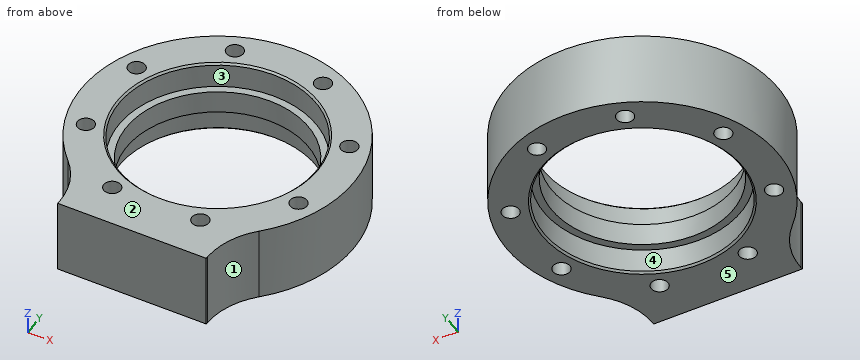
Autodesk Inventor part; units mm, degrees
ref_plane "YZ Plane" through (0, 0, 0) normal (1, 0, 0) x (0, 1, 0)
ref_plane "XZ Plane" through (0, 0, 0) normal (0, 1, 0) x (-1, 0, 0)
ref_plane "XY Plane" through (0, 0, 0) normal (0, 0, 1) x (1, 0, 0)
sketch "スケッチ1" plane through (0, 0, 0) normal (1, 0, 0) x (0, 1, 0)
  line L0 (26.1, 0) -> (36.1, 0)
  line L1 (36.1, 0) -> (36.1, 20)
  line L2 (36.1, 20) -> (26.1, 20)
  line L3 (26.1, 20) -> (26.1, 13.05)
  line L4 (26.1, 13.05) -> (24.1, 13.05)
  line L5 (0, -4) -> (0, 24)
  line L6 (24.1, 13.05) -> (24.1, 6.95)
  line L7 (24.1, 6.95) -> (26.1, 6.95)
  line L8 (26.1, 6.95) -> (26.1, 0)
  point P0 (0, 0)
  dimension "d0" = 26.1
  dimension "d2" = 6.95
  dimension "d3" = 20
  dimension "d4" = 10
  dimension "d28" = 2
  dimension "d29" = 6.95
revolve "回転1" add sketch "スケッチ1" angle 360 about axis through (0, 0, -10) along (0, 0, 1)
sketch "スケッチ2" plane through (0, 0, 0) normal (0, 0, -1) x (-1, 0, 0)
  circle A0 centre (0, 0) radius 31
  point P0 (-11.8632, 28.6403)
  point P1 (-28.6403, 11.8632)
  point P2 (-28.6403, -11.8632)
  point P3 (-11.8632, -28.6403)
  point P4 (11.8632, -28.6403)
  point P5 (28.6403, -11.8632)
  point P6 (28.6403, 11.8632)
  point P7 (11.8632, 28.6403)
  dimension "d6" = 62
  dimension "d9" = 360
  dimension "d25" = 0
hole "穴1" at (11.8632, 28.6403, 0) at (28.6403, 11.8632, 0) at (28.6403, -11.8632, 0) at (11.8632, -28.6403, 0) at (-11.8632, -28.6403, 0) at (-28.6403, -11.8632, 0) at (-28.6403, 11.8632, 0) at (-11.8632, 28.6403, 0) direction (0, 0, 1) diameter 4.5 end through all
chamfer "面取り1" distance 0.5 angle 45 2 edges at (0, -26.1, 20) (0, -26.1, 0)
sketch "スケッチ3" plane through (0, 0, 0) normal (0, 0, -1) x (-1, 0, 0)
  line L0 (-20, -30.0535) -> (20, -30.0535)
  line L1 (20, -30.0535) -> (20, -40)
  line L2 (20, -40) -> (-20, -40)
  line L3 (-20, -40) -> (-20, -30.0535)
  line L4 (-20, -30.0535) -> (20, -40) construction
  line L5 (20, -30.0535) -> (-20, -40) construction
  circle A0 centre (0, 0) radius 36.1
  point P0 (0, -35.0267)
  point P1 (0, -35.0267)
  point P2 (20, -30.0535)
  dimension "d21" = 40
  dimension "d22" = 40
extrude "押し出し1" add sketch "スケッチ3" against normal up to surface (20 mm away) contours A0 L1 L2 L3
fillet "フィレット2" radius 20 2 edges at (20, -30.0535, 10) (-20, -30.0535, 10)
ref_plane "作業平面1" through (-20, -40, 10) normal (0, 0, 1) x (1, 0, 0)
equation "\"d29\" = d2"
properties part number "scara-base15" material "ABS プラスチック"
Work out the finished part from the listing and answer in its coordinate system (mm). Face numbers are marked on the shaded views. A direction names the side the tool comes from. Round coordinates to 2 decimals unless told otherwise and drop trailing zeros. Loops run counter-clockwise (first coordinate to the right, second up) from the corner with the lowest first, then second, coordinate; pieces in that order, holes last.
(1) The mould has two halves that part along X. Classify the marked faces 1, 2 and 3: pulls with the +X half, pulls with the -X half, needs draft (parallel to the pull), parting line crosses it, or undercut.
Computed values:
face 1: pulls with the +X half
face 2: needs draft
face 3: undercut
(2) The part is cut by section A-A, the plane x = 0. Give the vertices of the cut face in (y, z), and give its area (3 significant figures).
Computed values:
outline: (-40, 0) - (-26.6, 0) - (-26.1, 0.5) - (-26.1, 6.95) - (-24.1, 6.95) - (-24.1, 13.05) - (-26.1, 13.05) - (-26.1, 19.5) - (-26.6, 20) - (-40, 20) - close; (24.1, 6.95) - (26.1, 6.95) - (26.1, 0.5) - (26.6, 0) - (36.1, 0) - (36.1, 20) - (26.6, 20) - (26.1, 19.5) - (26.1, 13.05) - (24.1, 13.05) - close
area: 502 mm2
(3) The part is cut by section B-B, the plane y = 0. Give the vertices of the cut face in (x, z).
Computed values:
outline: (-36.1, 0) - (-26.6, 0) - (-26.1, 0.5) - (-26.1, 6.95) - (-24.1, 6.95) - (-24.1, 13.05) - (-26.1, 13.05) - (-26.1, 19.5) - (-26.6, 20) - (-36.1, 20) - close; (24.1, 6.95) - (26.1, 6.95) - (26.1, 0.5) - (26.6, 0) - (36.1, 0) - (36.1, 20) - (26.6, 20) - (26.1, 19.5) - (26.1, 13.05) - (24.1, 13.05) - close
(4) For the marked faces 4 and 5, determine the directions among +Z, -Z, +X, -X, +Y, -Y from which every point of the face is accessible in a straight line to the end or side of a thin tool.
Computed values:
face 4: -Z
face 5: -Z, +X, -X, +Y, -Y
(5) Each of these flat-tipped pins is pushed along its axis until it touches: P1, Ø5, axis at x = -28.64, y = -11.86, coming from the -Z side; P2, Ø8, axis at y = -28, z = 15, coming from the +X side; P3, Ø4, axis at y = 12.5, z = 4, coming from the -X side; P4, Ø0.7, axis at y = -39.5, z = 14, coming from the -X side. Where does it stop, or does it pass through?
Computed values:
P1: stops at z = 0
P2: stops at x = 26.97
P3: stops at x = -34.54
P4: stops at x = -20
(6) Find the intervals of material crossed by L1, parallel to Y at x = 0, z = 5.25; L2, parallel to Y at x = 11, z = 19.25; L3, parallel to X at y = 29.5, z = 2, in increasing order.
Computed values:
L1: y = -40 to -26.1, 26.1 to 36.1
L2: y = -40 to -30.72, -26.56 to -23.67, 23.67 to 26.56, 30.72 to 34.38
L3: x = -20.81 to -13.94, -9.78 to 9.78, 13.94 to 20.81
(7) The part is cut by section C-C, the plane z = 10.5. Give the number of separate pieces and of enclosed holes in the cut face, and give its area (3 significant figures).
Computed values:
separate pieces: 1
enclosed holes: 9
area: 2,400 mm2
